```python
from build123d import *

# Parameters (mm, degrees)
SKETCH_1_W          = 15
SKETCH_1_H          = 15
SKETCH_1_W_2        = 12
SKETCH_1_H_2        = 12
EXTRUDE_1_DEPTH     = 135
SKETCH_2_R          = 2.7
CUT_EXTRUDE_1_DEPTH = 25
SKETCH_3_R          = 2.7
CUT_EXTRUDE_2_DEPTH = 25
SKETCH_5_R          = 5
CUT_EXTRUDE_4_DEPTH = 10


with BuildPart() as part:
    # ｽｹｯﾁ1 → ﾎﾞｽ - 押し出し1 (new body)
    with BuildSketch(Plane.XY):
        Rectangle(SKETCH_1_W, SKETCH_1_H)
        Rectangle(SKETCH_1_W_2, SKETCH_1_H_2, mode=Mode.SUBTRACT)
    extrude(amount=EXTRUDE_1_DEPTH)

    # ｽｹｯﾁ2 → ｶｯﾄ - 押し出し1 (cut)
    with BuildSketch(Plane(origin=(7.5, 0, 0), x_dir=(0, 0, -1), z_dir=(1, 0, 0))):
        with Locations((-112.5, 0)):
            Circle(SKETCH_2_R)
        with Locations((-22.5, 0)):
            Circle(SKETCH_2_R)
    extrude(amount=-CUT_EXTRUDE_1_DEPTH, mode=Mode.SUBTRACT)

    # ｽｹｯﾁ3 → ｶｯﾄ - 押し出し2 (cut)
    with BuildSketch(Plane(origin=(0, 7.5, 0), x_dir=(1, 0, 0), z_dir=(0, 1, 0))):
        with Locations((0, -7.5)):
            Circle(SKETCH_3_R)
        with Locations((0, -127.5)):
            Circle(SKETCH_3_R)
    extrude(amount=-CUT_EXTRUDE_2_DEPTH, mode=Mode.SUBTRACT)

    # ｽｹｯﾁ5 → ｶｯﾄ - 押し出し4 (cut)
    with BuildSketch(Plane(origin=(7.5, 0, 0), x_dir=(0, 0, -1), z_dir=(1, 0, 0))):
        with Locations((-22.5, 0)):
            Circle(SKETCH_5_R)
        with Locations((-112.5, 0)):
            Circle(SKETCH_5_R)
    extrude(amount=-CUT_EXTRUDE_4_DEPTH, mode=Mode.SUBTRACT)


solid = part.part
```
The model under review builds one solid part; all positions refer to its coordinate system, in mm. A direction names the side the tool comes from. Give positions to 0.01 mm unless a question says otherwise; leave off trailing zeros. Write each loop counter-clockwise with the first axis right and the second up, starting at its lowest first coordinate (ties: lowest second). Pieces come first, ordered by that corner, then holes. Notation, with made-up numbers: (19, -16.75) -> (29, -16.75) arc R14 cw to (29, 0.25) -> close; hole circle Ø2 at (22.5, 11.25). An arc over 180 degrees is marked (long way). Answer in a Markdown table with one row per item.
1) Add section B-B on y = 0. State the section outline as (x, z) points, plus the area to 3 significant figures.
Worked answers:
| item | result |
|---|---|
| outline | (-7.5, 0) -> (-6, 0) -> (-6, 19.8) -> (-7.5, 19.8) -> close; (-7.5, 25.2) -> (-6, 25.2) -> (-6, 109.8) -> (-7.5, 109.8) -> close; (-7.5, 115.2) -> (-6, 115.2) -> (-6, 135) -> (-7.5, 135) -> close; (6, 0) -> (7.5, 0) -> (7.5, 17.5) -> (6, 17.5) -> close; (6, 27.5) -> (7.5, 27.5) -> (7.5, 107.5) -> (6, 107.5) -> close; (6, 117.5) -> (7.5, 117.5) -> (7.5, 135) -> (6, 135) -> close |
| area | 359 mm² |
2) Add section A-A on x = 4.5. State the section outline as (y, z) points.
Worked answers:
| item | result |
|---|---|
| outline | (-7.5, 0) -> (-6, 0) -> (-6, 135) -> (-7.5, 135) -> close; (6, 0) -> (7.5, 0) -> (7.5, 135) -> (6, 135) -> close |
3) Mouldability with a two-part tool opening along Y and no side actions: class faces 1 (the cylindrical face through (-6.74, 2.277, 111.048)), 2 (the cylindrical face through (1.246, 6.76, 129.895)), 3 (the flat face through (0, -7.5, 67)) as +Y half, -Y half, draft (parallel to the pull), parting line (faces both ways), or undercut.
Worked answers:
| item | result |
|---|---|
| face 1 | undercut |
| face 2 | draft |
| face 3 | -Y half |
4) Add section C-C on z = 7.5. State the section outline as (x, y) points, plus the area to 3 significant figures.
Worked answers:
| item | result |
|---|---|
| outline | (-7.5, -7.5) -> (-2.7, -7.5) -> (-2.7, -6) -> (-6, -6) -> (-6, 6) -> (-2.7, 6) -> (-2.7, 7.5) -> (-7.5, 7.5) -> close; (2.7, -7.5) -> (7.5, -7.5) -> (7.5, 7.5) -> (2.7, 7.5) -> (2.7, 6) -> (6, 6) -> (6, -6) -> (2.7, -6) -> close |
| area | 64.8 mm² |
5) Add section D-D on z = 112.5. State the section outline as (x, y) points.
Worked answers:
| item | result |
|---|---|
| outline | (-7.5, -7.5) -> (7.5, -7.5) -> (7.5, -5) -> (6, -5) -> (6, -6) -> (-6, -6) -> (-6, -2.7) -> (-7.5, -2.7) -> close; (-7.5, 2.7) -> (-6, 2.7) -> (-6, 6) -> (6, 6) -> (6, 5) -> (7.5, 5) -> (7.5, 7.5) -> (-7.5, 7.5) -> close |
6) For L1, parallel to Y at x = 6.35, z = 22.5; L2, parallel to X at y = -7.05, z = 127.5; L3, parallel to Z at x = 0, y = 7, list the stretches that pass through material, from the lowest coordinate up. Write a range as [from, to].
Worked answers:
| item | result |
|---|---|
| L1 | [-7.5, -5], [5, 7.5] |
| L2 | [-7.5, -2.7], [2.7, 7.5] |
| L3 | [0, 4.8], [10.2, 124.8], [130.2, 135] |
7) Clearance check with a flat-ended pin moving along its axis: P1, Ø7, axis at y = 0, z = 22.5, coming from the +X side. State where the tip first meets the part, or that it passes through.
Worked answers:
| item | result |
|---|---|
| P1 | x = -6 |
8) Tool access review of faces 4 (the flat face through (6, 0, 67)), 5 (the cylindrical face through (6.76, -1.915, 107.881)), 6 (the cylindrical face through (1.246, -6.74, 129.895)): name each direction out of +Z, -Z, +X, -X, +Y, -Y from which nothing blocks a thin tool from reaching the whole face with its end or side.
Worked answers:
| item | result |
|---|---|
| face 4 | +Z, -Z |
| face 5 | +X |
| face 6 | +Y, -Y |
